Check sheet for the modelled part. Datum: model origin and axes. Units: mm. A direction names the side the tool comes from. Coordinates: 2 decimals unless noted, no trailing zeros. Loops run counter-clockwise (first coordinate to the right, second up) from the corner with the lowest first, then second, coordinate; pieces in that order, holes last. Notation, with made-up numbers: M 23,83 L 56,83 A22 cw 56,94 Z; hole C 76,-19 d9. An arc over 180 degrees is marked long. Use CSV: the item, a comma, the result in double quotes. Start each with the question number.
(1) Scan lines: line 1 (X direction, y = 22, z = 10); line 2 (X direction, y = 160.5, z = 5); line 3 (Y direction, x = -50, z = 39). Record each from-to range of solid material in increasing order.
(2) Section check A-A on z = 41.5. Record the cut outline in (x, y).
(3) Draft check along X on faces 1 (the flat face through (18, -30, 0)), 2 (the cylindrical face through (24.479, 264.332, 30.812)), 3 (the flat face through (-21, 204, 6.25)). Enter one of: pulls with the +X half, pulls with the -X half, needs draft (parallel to the pull), parting line crosses it, or undercut.
(4) Section check B-B on x = -47. Record the cut outline in (y, z), and give its area (3 significant figures).
(5) Section check D-D on x = -177. Record the cut outline in (y, z).
(6) Section check C-C on y = 49.5. Record the cut outline in (x, z).
(7) Go/stop test with flat-tipped pins: pin 1 Ø1.6 at (x, z) = (241, 30) entering from +Y; pin 2 Ø8 at (y, z) = (181.5, 50.5) entering from -X; pin 3 Ø10 at (y, z) = (1.5, 44) entering from +X. Record where each tip stops, or that it passes through.
(8) Set-up check for faces 4 (the flat face through (-116.045, 23, 31)), 5 (the flat face through (158.955, 20, 31)), 6 (the flat face through (-228.545, -178, 31)), 7 (the cylindrical face through (9.251, 219.818, 3.081)): record each of +Z, -Z, +X, -X, +Y, -Y from which the full face is reachable in a straight line by a thin tool's end or side.
from build123d import *

# Parameters (mm, degrees)
SKETCH1_R                                           = 87.5
BOSS_EXTRUDE1_DEPTH                                 = 62.5
FILLET1_R                                           = 50
SKETCH2_R                                           = 93.75
CUT_EXTRUDE3_DEPTH                                  = 6.25
CBORE_FOR_00_BINDING_HEAD_MACHINE_SCREW_D           = 1.397
CBORE_FOR_00_BINDING_HEAD_MACHINE_SCREW_CBORE_D     = 3.175
CBORE_FOR_00_BINDING_HEAD_MACHINE_SCREW_CBORE_DEPTH = 0.7112


with BuildPart() as part:
    # Sketch1 → Boss-Extrude1 (new body)
    with BuildSketch(Plane.XY):
        with BuildLine():
            Line((-228.544776119, -223.134328358), (271.455223881, -223.134328358))
            Line((271.455223881, -223.134328358), (271.455223881, -133.582089552))
            Line((271.455223881, -133.582089552), (158.955223881, -133.582089552))
            Line((158.955223881, -133.582089552), (158.955223881, 126.865671642))
            ThreePointArc((158.955223881, 126.865671642), (21.455223881, 264.365671642), (-116.044776119, 126.865671642))
            Line((-116.044776119, 126.865671642), (-116.044776119, -133.582089552))
            Line((-116.044776119, -133.582089552), (-228.544776119, -133.582089552))
            Line((-228.544776119, -133.582089552), (-228.544776119, -223.134328358))
        make_face()
        with Locations((21.455223881, 126.865671642)):
            Circle(SKETCH1_R, mode=Mode.SUBTRACT)
    extrude(amount=BOSS_EXTRUDE1_DEPTH)

    # Fillet1
    fillet1_edges = [part.edges().sort_by_distance(p)[0] for p in [
        (-116.044776119, -133.582089552, 31.25),
        (158.955223881, -133.582089552, 31.25),
    ]]
    fillet(fillet1_edges, radius=FILLET1_R)

    # Sketch2 → Cut-Extrude3 (cut)
    with BuildSketch(Plane.XY):
        with Locations((21.455223881, 126.865671642)):
            Circle(SKETCH2_R)
    extrude(amount=CUT_EXTRUDE3_DEPTH, mode=Mode.SUBTRACT)

    # CBORE for #00 Binding Head Machine Screw1 (through all)
    with Locations(Plane(origin=(0, -133.582089552, 0), x_dir=(1, 0, 0), z_dir=(0, 1, 0))):
        with Locations((-198.798502654, -30.325345844), (240.412221484, -30.325345844)):
            CounterBoreHole(CBORE_FOR_00_BINDING_HEAD_MACHINE_SCREW_D / 2, CBORE_FOR_00_BINDING_HEAD_MACHINE_SCREW_CBORE_D / 2, CBORE_FOR_00_BINDING_HEAD_MACHINE_SCREW_CBORE_DEPTH)


solid = part.part
Outcome:
1,line 1,"x = -116.04 to 158.96"
1,line 2,"x = -111.87 to -66.05, 108.96 to 154.78"
1,line 3,"y = -223.13 to 76.36, 177.37 to 244.34"
2,outline,"M -228.54,-223.13 L 271.46,-223.13 L 271.46,-133.58 L 208.96,-133.58 A50 cw 158.96,-83.58 L 158.96,126.87 A137.5 ccw -116.04,126.87 L -116.04,-83.58 A50 cw -166.04,-133.58 L -228.54,-133.58 Z; hole C 21.46,126.87 d175"
3,face 1,"needs draft"
3,face 2,"parting line crosses it"
3,face 3,"undercut"
4,outline,"M -223.13,0 L 62.81,0 L 62.81,6.25 L 72.37,6.25 L 72.37,62.5 L -223.13,62.5 Z; M 181.36,6.25 L 190.92,6.25 L 190.92,0 L 246.11,0 L 246.11,62.5 L 181.36,62.5 Z"
4,area,"22,400 mm²"
5,outline,"M -223.13,0 L -133.58,0 L -133.58,62.5 L -223.13,62.5 Z"
6,outline,"M -116.04,0 L -31.49,0 L -31.49,6.25 L -19.42,6.25 L -19.42,62.5 L -116.04,62.5 Z; M 62.33,6.25 L 74.4,6.25 L 74.4,0 L 158.96,0 L 158.96,62.5 L 62.33,62.5 Z"
7,pin 1,"stops at y = -134.29"
7,pin 2,"stops at x = -106.38"
7,pin 3,"stops at x = 158.96"
8,face 4,"+Z, -Z, -X, +Y"
8,face 5,"+Z, -Z, +X, +Y"
8,face 6,"+Z, -Z, -X, +Y, -Y"
8,face 7,"-Z"
